Could you check a few things on this model? Use its own coordinates, in mm. Coordinates: 2 decimals unless noted, no trailing zeros. Order: outer loops, then holes, each group sorted by start corner. A loop starts at its lowest first (then second) coordinate and runs counter-clockwise, first axis right, second up. Notation, with made-up numbers: (46.25, 0.25) - (89.25, 0.25) arc R17 cw to (89.25, 4.25) - close; hole circle Ø6 at (52, 7.25). An arc over 180 degrees is marked (long way). Answer as CSV lines item,"result". Start each with the question number.
1. I want a section at B-B, the plane x = -21.5. List the corners of the cut face in (y, z) for me, and give its area (3 significant figures).
2. I want a section at A-A, the plane y = 0. List the corners of the cut face in (x, z) for me.
3. I want a section at C-C, the plane z = 23.5. List the corners of the cut face in (x, y) for me.
4. I need wall thicknesses on probe 1 along Y at (x, z) = (0, 7.75); probe 2 along X at (y, z) = (0.5, 24); probe 3 along Y at (x, z) = (-1.5, 19.75). Which ranges of each line are inside material? Lowest first, please.
5. For pin 1 (4 mm diameter, centred on x = -9, z = 11.5, fed in from +Y); pin 2 (3 mm diameter, centred on x = 13, z = 15, fed in from -Y); pin 3 (10 mm diameter, centred on x = -34.5, z = 5, fed in from +Y); pin 4 (12 mm diameter, centred on y = 27, z = 9, fed in from -X), each with a flat end and sliding along its axis, tell me the tip position at first contact or that it passes through.
6. I want a section at D-D, the plane z = 2.75. List the corners of the cut face in (x, y) for me, and give its area (3 significant figures).
7. Thinking about a two-plate mould opening in X: for faces 1 (the face through (-6.326, -28.488, 12.878)), 2 (the face through (22.7, -40.1, 12.5)), 3 (the face through (-1, -31, 0)), which applies, released by +X, released by -X, zero draft, split by the parting line, or undercut?
from build123d import *

# Parameters (mm, degrees)
F1_DEPTH = 25.4
F2_R     = 29.1814766443
F3_DEPTH = 25.4


with BuildPart() as f1:
    # F0 (on Top) → F1 (new body)
    with BuildSketch(Plane.XY):
        Polygon((46.0779853165, -26.6031372262), (46.0779853165, 26.6031372262), (0, 53.2062744524), (-46.0779853165, 26.6031372262), (-46.0779853165, -26.6031372262), (0, -53.2062744524), align=None)
    extrude(amount=F1_DEPTH)

    # F2 (on face) → F3 (cut)
    with BuildSketch(Plane.XY.offset(25.4)):
        Circle(F2_R)
    extrude(amount=-F3_DEPTH, mode=Mode.SUBTRACT)

    # F4 (on Right) → F5 (revolve, cut)
    with BuildSketch(Plane.YZ):
        with BuildLine():
            Line((53.2062744524, 25.4), (46.8562744524, 25.4))
            ThreePointArc((46.8562744524, 25.4), (51.3464025129, 23.5401280605), (53.2062744524, 19.05))
            Line((53.2062744524, 19.05), (53.2062744524, 25.4))
        make_face()
    revolve(axis=Axis((0, 0, 25.4), (0, 0, 1)), mode=Mode.SUBTRACT)

    # F6 (on Right) → F7 (revolve, cut)
    with BuildSketch(Plane.YZ):
        with BuildLine():
            Line((53.2062744524, 0), (53.2062744524, 6.35))
            ThreePointArc((53.2062744524, 6.35), (51.3464025129, 1.8598719395), (46.8562744524, 0))
            Line((46.8562744524, 0), (53.2062744524, 0))
        make_face()
    revolve(axis=Axis((0, 0, 25.4), (0, 0, 1)), mode=Mode.SUBTRACT)


solid = f1.part
Solved:
1,outline,"(-40.79, 0) - (-19.73, 0) - (-19.73, 25.4) - (-40.79, 25.4) - close; (19.73, 0) - (40.79, 0) - (40.79, 25.4) - (19.73, 25.4) - close"
1,area,"1,070 mm2"
2,outline,"(-46.08, 0) - (-29.18, 0) - (-29.18, 25.4) - (-46.08, 25.4) - close; (29.18, 0) - (46.08, 0) - (46.08, 25.4) - (29.18, 25.4) - close"
3,outline,"(-46.08, -22.75) arc R51.39 ccw to (-42.74, -28.53) - (-3.34, -51.28) arc R51.39 ccw to (3.34, -51.28) - (42.74, -28.53) arc R51.39 ccw to (46.08, -22.75) - (46.08, 22.75) arc R51.39 ccw to (42.74, 28.53) - (3.34, 51.28) arc R51.39 ccw to (-3.34, 51.28) - (-42.74, 28.53) arc R51.39 ccw to (-46.08, 22.75) - close; hole circle Ø58.36 at (0, 0)"
4,probe 1,"y = -53.21 to -29.18, 29.18 to 53.21"
4,probe 2,"x = -46.08 to -29.18, 29.18 to 46.08"
4,probe 3,"y = -52.34 to -29.14, 29.14 to 52.34"
5,pin 1,"stops at y = 49.16"
5,pin 2,"stops at y = -46.57"
5,pin 3,"stops at y = 36.17"
5,pin 4,"stops at x = -46.08"
6,outline,"(-46.08, -24.29) arc R52.09 ccw to (-44.07, -27.76) - (-2.01, -52.05) arc R52.09 ccw to (2.01, -52.05) - (44.07, -27.76) arc R52.09 ccw to (46.08, -24.29) - (46.08, 24.29) arc R52.09 ccw to (44.07, 27.76) - (2.01, 52.05) arc R52.09 ccw to (-2.01, 52.05) - (-44.07, 27.76) arc R52.09 ccw to (-46.08, 24.29) - close; hole circle Ø58.36 at (0, 0)"
6,area,"4,670 mm2"
7,face 1,"undercut"
7,face 2,"released by +X"
7,face 3,"zero draft"
